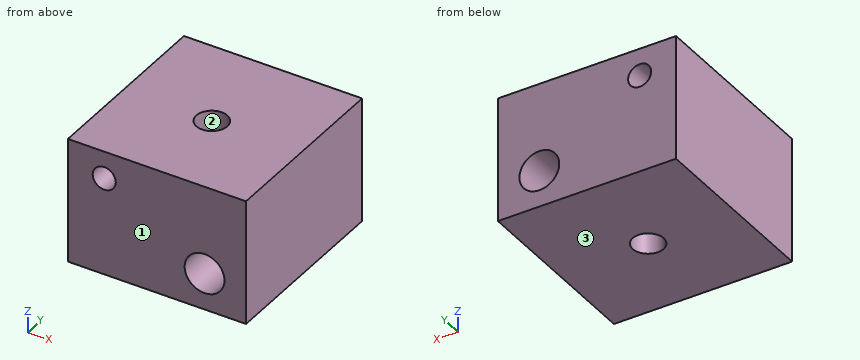
from build123d import *

# Parameters (mm, degrees)
F0_W          = 98.013702
F0_H          = 68.835622
F0_R          = 10.97537
F0_R_2        = 6.35
F1_DEPTH      = 63.5
F1_DEPTH_BACK = 38.1
F2_R          = 8.54279
F3_DEPTH      = 68.836623


with BuildPart() as f1:
    # F0 (on Front) → F1 (new body, two sides)
    with BuildSketch(Plane.XZ) as f1_sk:
        with Locations((5.161934, 2.408902)):
            Rectangle(F0_W, F0_H)
        with Locations((31.360572, -11.87192)):
            Circle(F0_R, mode=Mode.SUBTRACT)
        with Locations((-23.844917, 21.826713)):
            Circle(F0_R_2, mode=Mode.SUBTRACT)
    extrude(amount=F1_DEPTH)
    extrude(f1_sk.sketch, amount=-F1_DEPTH_BACK)

    # F2 (on face) → F3 (cut, through all)
    with BuildSketch(Plane.XY.offset(36.826713)):
        with Locations((4.90384, -15.055645)):
            Circle(F2_R)
    extrude(amount=-F3_DEPTH, mode=Mode.SUBTRACT)


solid = f1.part
CAD build for the part. Positions are in the model's coordinates, mm. Face numbers are marked on the shaded views. Coordinates: 2 decimals unless noted, no trailing zeros. Order: outer loops, then holes, each group sorted by start corner. A loop starts at its lowest first (then second) coordinate and runs counter-clockwise, first axis right, second up. Notation, with made-up numbers: (10.5, -3) -> (51.5, -3) arc R20 ccw to (51.5, 10) -> close; hole circle Ø1 at (83.5, 4). An arc over 180 degrees is marked (long way). Answer in a Markdown table with one row per item.
1) Mould opens along Y. For the marked faces 1, 2 and 3 say: pulls with the +Y half, pulls with the -Y half, needs draft (parallel to the pull), parting line crosses it, or undercut.
Check values:
| item | result |
|---|---|
| face 1 | pulls with the -Y half |
| face 2 | undercut |
| face 3 | needs draft |
2) Band-saw the part on A-A (z = -13.5). List the corners of the cut face in (x, y), and give its area (3 significant figures).
Check values:
| item | result |
|---|---|
| outline | (-43.84, -63.5) -> (20.51, -63.5) -> (20.51, 38.1) -> (-43.84, 38.1) -> close; (42.21, -63.5) -> (54.17, -63.5) -> (54.17, 38.1) -> (42.21, 38.1) -> close; hole circle Ø17.09 at (4.9, -15.06) |
| area | 7,520 mm2 |
3) Band-saw the part on B-B (x = 38). List the corners of the cut face in (y, z).
Check values:
| item | result |
|---|---|
| outline | (-63.5, -32.01) -> (38.1, -32.01) -> (38.1, -20.61) -> (-63.5, -20.61) -> close; (-63.5, -3.13) -> (38.1, -3.13) -> (38.1, 36.83) -> (-63.5, 36.83) -> close |
4) Drill centre lines: line 1 (Z direction, x = 28, y = -2); line 2 (Z direction, x = -22.5, y = 12); line 3 (Y direction, x = 0.5, z = -15.5). Where is each one in solid material? Low to high.
Check values:
| item | result |
|---|---|
| line 1 | -32.01 to -22.32, -1.42 to 36.83 |
| line 2 | -32.01 to 15.62, 28.03 to 36.83 |
| line 3 | -63.5 to -22.38, -7.74 to 38.1 |
5) Band-saw the part on D-D (y = 11.5). List the corners of the cut face in (x, z).
Check values:
| item | result |
|---|---|
| outline | (-43.84, -32.01) -> (54.17, -32.01) -> (54.17, 36.83) -> (-43.84, 36.83) -> close; hole circle Ø12.7 at (-23.84, 21.83); hole circle Ø21.95 at (31.36, -11.87) |
6) Band-saw the part on C-C (z = 17). List the corners of the cut face in (x, y), and give its area (3 significant figures).
Check values:
| item | result |
|---|---|
| outline | (-43.84, -63.5) -> (-27.97, -63.5) -> (-27.97, 38.1) -> (-43.84, 38.1) -> close; (-19.72, -63.5) -> (54.17, -63.5) -> (54.17, 38.1) -> (-19.72, 38.1) -> close; hole circle Ø17.09 at (4.9, -15.06) |
| area | 8,890 mm2 |
